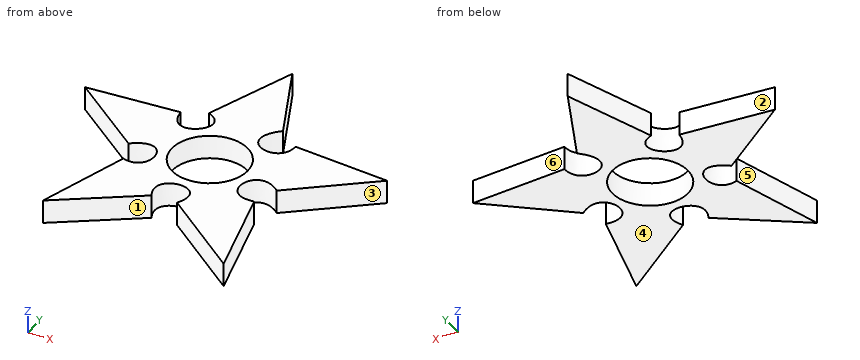
from build123d import *

# Parameters (mm, degrees)
F0_R     = 11.25
F1_DEPTH = 7


with BuildPart() as f1:
    # F0 (on Top) → F1 (new body)
    with BuildSketch(Plane.XY):
        with BuildLine():
            Line((3.053512, 35.332328), (-6.700666, 8.404746))
            add(Edge.make_bspline(
                [(-13.344336, 5.164926), (-12.019685, -7.597877), (3.565281, 4.258171), (-6.700666, 8.404746)],
                knots=[0, 0, 0, 0, 7.391535, 7.391535, 7.391535, 7.391535], degree=3))
            Line((-13.344336, 5.164926), (-40.870471, 3.228944))
            Line((-40.870471, 3.228944), (-17.937381, -14.382361))
            add(Edge.make_bspline(
                [(-17.937381, -14.382361), (-7.205485, -5.840566), (-5.676269, -24.48345), (-15.58056, -21.261975)],
                knots=[0, 0, 0, 0, 7.272117, 7.272117, 7.272117, 7.272117], degree=3))
            Line((-15.58056, -21.261975), (-24.037964, -48.886847))
            Line((-24.037964, -48.886847), (-0.577154, -32.873667))
            add(Edge.make_bspline(
                [(-0.577154, -32.873667), (-6.186889, -22.709077), (12.788273, -21.840621), (6.892902, -32.576927)],
                knots=[0, 0, 0, 0, 7.475948, 7.475948, 7.475948, 7.475948], degree=3))
            Line((6.892902, -32.576927), (31.716839, -51.809535))
            Line((31.716839, -51.809535), (24.148522, -22.221368))
            add(Edge.make_bspline(
                [(24.148522, -22.221368), (12.527963, -23.872861), (17.102542, -6.313425), (26.725877, -14.832847)],
                knots=[0, 0, 0, 0, 7.825152, 7.825152, 7.825152, 7.825152], degree=3))
            Line((26.725877, -14.832847), (49.450749, 3.405918))
            Line((49.450749, 3.405918), (20.766794, 5.689487))
            add(Edge.make_bspline(
                [(14.262746, 10.579666), (3.641411, 0.945837), (20.901213, -4.688121), (20.766794, 5.689487)],
                knots=[0, 0, 0, 0, 8.137351, 8.137351, 8.137351, 8.137351], degree=3))
            Line((14.262746, 10.579666), (3.053512, 35.332328))
        make_face()
        with Locations((4.293832, -10.60445)):
            Circle(F0_R, mode=Mode.SUBTRACT)
    extrude(amount=F1_DEPTH)


solid = f1.part
Input: part model. Units: mm. Frame: model coordinates. Face numbers are marked on the shaded views. A direction names the side the tool comes from. Coordinates: 2 decimals unless noted, no trailing zeros. Loops run counter-clockwise (first coordinate to the right, second up) from the corner with the lowest first, then second, coordinate; pieces in that order, holes last. Notation, with made-up numbers: (73.5, -27) -> (99.5, -27) arc R25 ccw to (99.5, 5) -> close; hole circle Ø7 at (59.25, 41.25). An arc over 180 degrees is marked (long way). One line per item, written item: value.
(1) Pin query (flat end, axial travel): pin 1 Ø3 at (x, z) = (-31.5, 6) entering from +Y; pin 2 Ø1 at (x, z) = (-8.5, 3.5) entering from +Y; pin 3 Ø3 at (y, z) = (-14.5, 6) entering from -X. Return the tip coordinate at first contact, or that it passes through.
Answer below:
pin 1: stops at y = 3.99
pin 2: stops at y = -0.52
pin 3: stops at x = -19.74
(2) Draft query along Y for the marked faces 1, 2, 3 and 4. Return one class per face: pulls with the +Y half, pulls with the -Y half, needs draft (parallel to the pull), parting line crosses it, or undercut.
Answer below:
face 1: pulls with the -Y half
face 2: pulls with the +Y half
face 3: undercut
face 4: needs draft
(3) Set-up query: the marked faces 5 and 6. Return all of +Z, -Z, +X, -X, +Y, -Y with unobstructed straight access to the full face (end or side cutting, diameter ignored); none if empty.
Answer below:
face 5: +Z, -Z, -X
face 6: +Z, -Z, +X, +Y
(4) Cut plane A-A (x = -19). Output: boundary loops of the cut face in (y, z).
Answer below:
outline: (-45.45, 0) -> (-32.43, 0) -> (-32.43, 7) -> (-45.45, 7) -> close; (-13.57, 0) -> (4.77, 0) -> (4.77, 7) -> (-13.57, 7) -> close
(5) Ray query, line 1 along X through (y, z) = (-13.5, 6); line 2 along X through (y, z) = (-29, 4.5); line 3 along Y through (x, z) = (6, 2.25). Return the intervals inside material, ascending.
Answer below:
line 1: x = -19.09 to -16.72, -9.98 to -6.58, 15.16 to 18.99, 24.93 to 28.39
line 2: x = -17.95 to -1.61, 8.04 to 25.88
line 3: y = -25.44 to -21.72, 0.52 to 28.83
(6) Cut plane D-D (y = 15). Output: boundary loops of the cut face in (x, z).
Answer below:
outline: (-4.31, 0) -> (12.26, 0) -> (12.26, 7) -> (-4.31, 7) -> close
(7) Cut plane C-C (x = 38.5). Output: boundary loops of the cut face in (y, z), then the cut area to 3 significant figures.
Answer below:
outline: (-5.38, 0) -> (4.28, 0) -> (4.28, 7) -> (-5.38, 7) -> close
area: 67.6 mm2
(8) Cut plane B-B (y = -41.5). Output: boundary loops of the cut face in (x, z).
Answer below:
outline: (-21.78, 0) -> (-13.22, 0) -> (-13.22, 7) -> (-21.78, 7) -> close; (18.41, 0) -> (29.08, 0) -> (29.08, 7) -> (18.41, 7) -> close
